Geometry check sheet. Reference: the model listing, model coordinates, mm. Coordinates: 2 decimals unless noted, no trailing zeros. Write each loop counter-clockwise with the first axis right and the second up, starting at its lowest first coordinate (ties: lowest second). Pieces come first, ordered by that corner, then holes. Notation, with made-up numbers: M -6,-32 L 11,-32 A24 cw 11,-21 Z; hole C -5.75,89 d10. An arc over 180 degrees is marked long. Put each result on its own line as item: value. Start each with the question number.
1) Cross-section at B-B on z = 0. Record the cut outline in (x, y).
2) Scan lines: line 1 along Y through (x, z) = (-0.15, 0); line 2 along Z through (x, y) = (2, 1.6); line 3 along X through (y, z) = (0.2, 0.35). Record each from-to range of solid material in increasing order.
3) Mould release check, pull along Z, two halves, no side actions. Record for faces 1 (the flat face through (0, 2, -2.5)), 2 (the flat face through (-3.5, 3, 1)), 3 (the cylindrical face through (-0.042, 2.373, -0.104)), 4 (the flat face through (0, 2, 2.5)): released by +Z, released by -Z, zero draft, split by the parting line, or undercut.
4) Cross-section at D-D on z = -2.05. Record the cut outline in (x, y).
5) Gauge pin test, flat end, axial feed: pin 1 (1.3 mm diameter, centred on y = 1.58, z = 0, fed in from -X). Record the tip position at first contact, or that the pin passes through.
6) Cross-section at A-A on y = 1.58. Record the cut outline in (x, z), plus the area to 3 significant figures.
7) Cross-section at C-C on x = 2. Record the cut outline in (y, z), plus the area to 3 significant figures.
from build123d import *

# Parameters (mm, degrees)
SKETCH1_W           = 6
SKETCH1_H           = 5
BOSS_EXTRUDE1_DEPTH = 0.5
SKETCH2_W           = 7
SKETCH2_H           = 5
BOSS_EXTRUDE2_DEPTH = 2.66
SKETCH3_R           = 0.8
CUT_EXTRUDE1_DEPTH  = 9.076855824
CHAMFER1_SIZE       = 0.5


with BuildPart() as part:
    # Sketch1 → Boss-Extrude1 (new body)
    with BuildSketch(Plane(origin=(0, 0, 0), x_dir=(1, 0, 0), z_dir=(0, 1, 0))):
        Rectangle(SKETCH1_W, SKETCH1_H)
    extrude(amount=BOSS_EXTRUDE1_DEPTH)

    # Sketch2 → Boss-Extrude2 (add)
    with BuildSketch(Plane(origin=(0, 0.5, 0), x_dir=(1, 0, 0), z_dir=(0, 1, 0))):
        Rectangle(SKETCH2_W, SKETCH2_H)
    extrude(amount=BOSS_EXTRUDE2_DEPTH)

    # Sketch3 → Cut-Extrude1 (cut, through all)
    with BuildSketch(Plane.ZY.offset(3.5)):
        with Locations((0, 1.58)):
            Circle(SKETCH3_R)
    extrude(amount=-CUT_EXTRUDE1_DEPTH, mode=Mode.SUBTRACT)

    # Chamfer1
    # the kernel refuses this chamfer: 0.5 mm, written as the material it takes off along each edge
    with BuildSketch(Plane(origin=(3.5, 1.58, 0), x_dir=(0, 0, 1), z_dir=(0, -1, 0))) as chamfer1_piece_1:
        Polygon((0.8 + CHAMFER1_SIZE, 0), (0.8, CHAMFER1_SIZE), (0.8, 0), align=None)
    revolve(axis=Axis((3.5, 1.58, 0), (-1, 0, 0)), mode=Mode.SUBTRACT)
    with BuildSketch(Plane(origin=(-3.5, 1.58, 0), x_dir=(0, 0, 1), z_dir=(0, -1, 0))) as chamfer1_piece_2:
        Polygon((0.8 + CHAMFER1_SIZE, 0), (0.8, -CHAMFER1_SIZE), (0.8, 0), align=None)
    revolve(axis=Axis((-3.5, 1.58, 0), (-1, 0, 0)), mode=Mode.SUBTRACT)


solid = part.part
Answer key:
1. outline: M -3.5,2.88 L -3,2.38 L 3,2.38 L 3.5,2.88 L 3.5,3.16 L -3.5,3.16 Z; M -3.28,0.5 L -3,0.5 L -3,0 L 3,0 L 3,0.5 L 3.28,0.5 L 3,0.78 L -3,0.78 Z
2. line 1: y = 0 to 0.78, 2.38 to 3.16
2. line 2: z = -2.5 to -0.8, 0.8 to 2.5
2. line 3: x = -3 to 3
3. face 1: released by -Z
3. face 2: zero draft
3. face 3: undercut
3. face 4: released by +Z
4. outline: M -3.5,0.5 L -3,0.5 L -3,0 L 3,0 L 3,0.5 L 3.5,0.5 L 3.5,3.16 L -3.5,3.16 Z
5. pin 1: passes through
6. outline: M -3.5,-2.5 L 3.5,-2.5 L 3.5,-1.3 L 3,-0.8 L -3,-0.8 L -3.5,-1.3 Z; M -3.5,1.3 L -3,0.8 L 3,0.8 L 3.5,1.3 L 3.5,2.5 L -3.5,2.5 Z
6. area: 23.3 mm²
7. outline: M 0,-2.5 L 3.16,-2.5 L 3.16,2.5 L 0,2.5 Z; hole C 1.58,0 d1.6
7. area: 13.8 mm²
